Here's the drawing with two shaded views (mm, measured from the low corner). I have some questions. A direction names the side the tool comes from. Round coordinates to 2 decimals unless told otherwise and drop trailing zeros. Loops run counter-clockwise (first coordinate to the right, second up) from the corner with the lowest first, then second, coordinate; pieces in that order, holes last.
(1) I want a section at B-B on x = 17.5. Write out the boundary of the cut face in (y, z), plus the area to 3 significant figures.
(2) I want a section at C-C on z = 5.5. Write out the boundary of the cut face in (x, y) (1 decimal).
(3) Will these pins go through, and if not, where does the flat tip stop? pin 1 Ø6 at (x, z) = (17, 5.5) entering from +Y; pin 2 Ø4 at (y, z) = (12.5, 5) entering from +X; pin 3 Ø3 at (y, z) = (14, 5.5) entering from +X.
(4) If I drill on line 1 along X through (y, z) = (1.4, 5); line 2 along Y through (x, z) = (0.75, 5); line 3 along Z through (x, y) = (17.5, 0.85), over which ranges is the centre line in solid material (lowest first)?
(5) I want a section at D-D on x = 8.5. Write out the boundary of the cut face in (y, z), plus the area to 3 significant figures.
(6) Which directions (+Z, -Z, +X, -X, +Y, -Y) give clear straight access to the entire face, cutting with the end or side of a thin tool? Please do the marked faces 5 and 6.
(7) I want a section at A-A on y = 12.5. Write out the boundary of the cut face in (x, z), plus the area to 3 significant figures.
(8) Thinking about a two-plate mould opening in X: for the marked faces 1, 2, 3 and 4, which applies, released by +X, released by -X, zero draft, split by the parting line, or undercut?
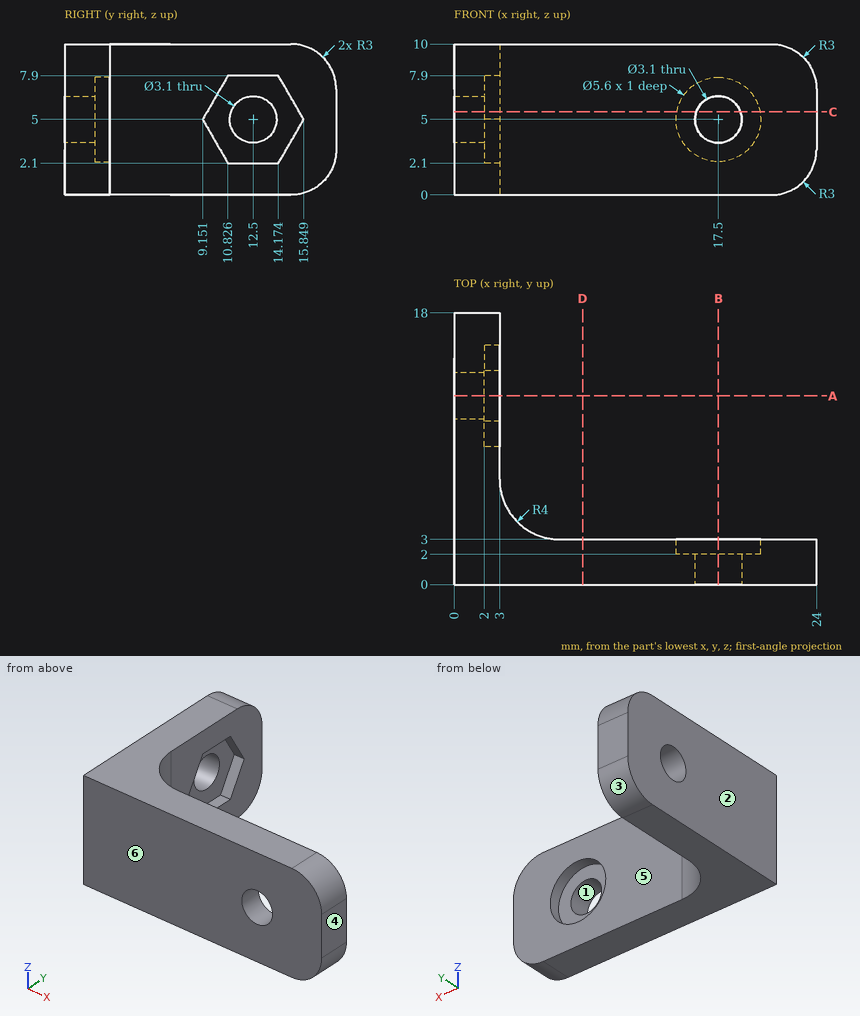
Filled sheet:
1. outline: (0, 0) - (3, 0) - (3, 2.2) - (2, 2.2) - (2, 3.45) - (0, 3.45) - close; (0, 6.55) - (2, 6.55) - (2, 7.8) - (3, 7.8) - (3, 10) - (0, 10) - close
1. area: 18.2 mm2
2. outline: (0, 0) - (16, 0) - (16, 2) - (14.7, 2) - (14.7, 3) - (7, 3) arc R4 cw to (3, 7) - (3, 9.4) - (2, 9.4) - (2, 11) - (0, 11) - close; (0, 14) - (2, 14) - (2, 15.6) - (3, 15.6) - (3, 18) - (0, 18) - close; (19, 0) - (24, 0) - (24, 3) - (20.3, 3) - (20.3, 2) - (19, 2) - close
3. pin 1: stops at y = 3
3. pin 2: stops at x = 2
3. pin 3: stops at x = 3
4. line 1: x = 0 to 15.95, 19.05 to 24
4. line 2: y = 0 to 10.95, 14.05 to 18
4. line 3: z = 0 to 3.45, 6.55 to 10
5. outline: (0, 0) - (3, 0) - (3, 10) - (0, 10) - close
5. area: 30.0 mm2
6. face 5: +Z, -Z, +X, +Y
6. face 6: +Z, -Z, +X, -X, -Y
7. outline: (0, 0) - (3, 0) - (3, 2.1) - (2, 2.1) - (2, 3.45) - (0, 3.45) - close; (0, 6.55) - (2, 6.55) - (2, 7.9) - (3, 7.9) - (3, 10) - (0, 10) - close
7. area: 18.0 mm2
8. face 1: undercut
8. face 2: released by -X
8. face 3: zero draft
8. face 4: released by +X
